Read the model definition and answer for the solid it produces. Units are mm, in the model's axes. Face numbers are marked on the shaded views. A direction names the side the tool comes from. Round coordinates to 2 decimals unless told otherwise and drop trailing zeros. Order: outer loops, then holes, each group sorted by start corner. A loop starts at its lowest first (then second) coordinate and runs counter-clockwise, first axis right, second up. Notation, with made-up numbers: (14, -24.5) -> (40, -24.5) arc R12 ccw to (40, -18.5) -> close; hole circle Ø11 at (61.25, 62). An arc over 180 degrees is marked (long way). Use a Markdown table: item, result. Add a question column.
1. For the marked faces 1 and 2, determine the directions among +Z, -Z, +X, -X, +Y, -Y from which every point of the face is accessible in a straight line to the end or side of a thin tool.
2. The mould has two halves that part along Y. Classify the marked faces 3, 4 and 5: +Y half, -Y half, draft (parallel to the pull), parting line (faces both ways), or undercut.
3. Section D-D, the plane x = -34.5 is taken. Give the vertices of the cut face in (y, z).
4. Section C-C, the plane x = -25.75 is taken. Give the vertices of the cut face in (y, z), then the cut area to 3 significant figures.
5. Given pin 1 (3 mm diameter, centred on x = -25.5, z = 389.5, fed in from -Y); pin 2 (8 mm diameter, centred on y = 15.27, z = 391.14, fed in from +X); pin 3 (6 mm diameter, centred on x = -28.5, z = 394.5, fed in from +Y); pin 4 (12 mm diameter, centred on x = -32, y = 17, fed in from +Z), each flat-ended and moving along its own axis, determine where each tip first touches the part or whether it passes through.
6. Section A-A, the plane y = 15.25 is taken. Give the vertices of the cut face in (x, z), then the cut area to 3 significant figures.
7. Section B-B, the plane z = 396 is taken. Give the vertices of the cut face in (x, y), then the cut area to 3 significant figures.
8. Consider L1, parallel to X at y = 12.75, z = 396.5; L2, parallel to Y at x = -22, z = 398.5; L3, parallel to Y at x = -36.75, z = 389.25. Determine where each line is inside the solid, lowest interval first. Write a range as [from, to].
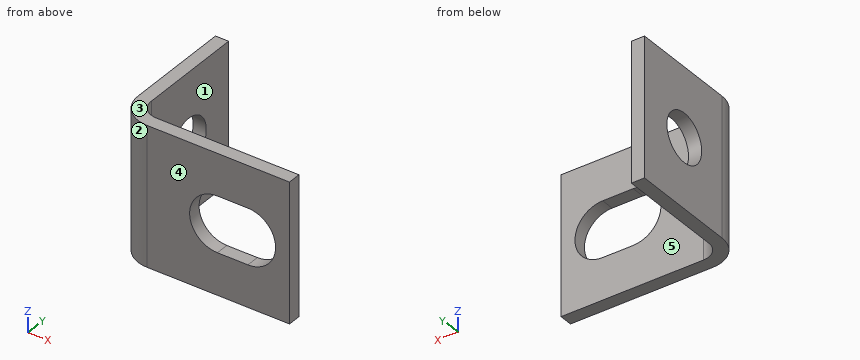
```python
from build123d import *

# Parameters (mm, degrees)
SKETCH2_W                    = 25
SKETCH2_H                    = 20
BASE_FLANGE1_DEPTH           = 1.89738
EDGE_FLANGE1_STRIP_W         = 12.66952
EDGE_FLANGE1_STRIP_H         = 1.89738
EDGE_FLANGE1_STRIP_CUT_DEPTH = 20
EDGE_FLANGE1_DEPTH           = 20
SKETCH11_R                   = 3.5
CUT_EXTRUDE1_DEPTH           = 10
CUT_EXTRUDE2_DEPTH           = 10


# Sheet-metal steps are written as plain solids
with BuildPart() as part:
    # Sketch2 → Base-Flange1 (new body)
    with BuildSketch(Plane(origin=(0, 3.26937922, 0), x_dir=(1, 0, 0), z_dir=(0, 1, 0))):
        with Locations((-25.783324161, -391.136685208)):
            Rectangle(SKETCH2_W, SKETCH2_H)
    extrude(amount=BASE_FLANGE1_DEPTH)

    # Edge-Flange1 strip (across the edge) → Edge-Flange1 strip cut (cut)
    with BuildSketch(Plane(origin=(-38.283324161, 5.16675922, 381.136685208), x_dir=(1, 0, 0), z_dir=(0, 0, 1))):
        with Locations((-1.89738, -0.94869)):
            Rectangle(EDGE_FLANGE1_STRIP_W, EDGE_FLANGE1_STRIP_H)
    extrude(amount=EDGE_FLANGE1_STRIP_CUT_DEPTH, mode=Mode.SUBTRACT)

    # Edge-Flange1 section (across the edge) → Edge-Flange1 (add)
    with BuildSketch(Plane(origin=(-38.283324161, 5.16675922, 381.136685208), x_dir=(1, 0, 0), z_dir=(0, 0, 1))):
        with BuildLine():
            Line((0, 2.54), (0, 18.10262))
            Line((0, 18.10262), (1.89738, 18.10262))
            Line((1.89738, 18.10262), (1.89738, 2.54))
            ThreePointArc((1.89738, 2.54), (2.641328776, 0.743948776), (4.43738, 0))
            Line((4.43738, 0), (4.43738, -1.89738))
            ThreePointArc((4.43738, -1.89738), (1.299678511, -0.597701489), (0, 2.54))
        make_face()
    extrude(amount=EDGE_FLANGE1_DEPTH)

    # Sketch11 → Cut-Extrude1 (cut)
    with BuildSketch(Plane.ZY.offset(38.283324161)):
        with Locations(Location((391.136685208, 15.26937922, 0), (0, 0, 270))):
            Circle(SKETCH11_R)
    extrude(amount=-CUT_EXTRUDE1_DEPTH, mode=Mode.SUBTRACT)

    # Sketch13 → Cut-Extrude2 (cut)
    with BuildSketch(Plane(origin=(0, 5.16675922, 0), x_dir=(1, 0, 0), z_dir=(0, 1, 0))):
        with BuildLine():
            Line((-23.678800395, -387.136685208), (-19.283324161, -387.136685208))
            ThreePointArc((-19.283324161, -387.136685208), (-15.283324161, -391.136685208), (-19.283324161, -395.136685208))
            Line((-19.283324161, -395.136685208), (-23.678800395, -395.136685208))
            ThreePointArc((-23.678800395, -395.136685208), (-27.678800395, -391.136685208), (-23.678800395, -387.136685208))
        make_face()
    extrude(amount=-CUT_EXTRUDE2_DEPTH, mode=Mode.SUBTRACT)


solid = part.part
```
Verdict:
| question | item | result |
|---|---|---|
| 1 | face 1 | +Z, -Z, +X, +Y |
| 1 | face 2 | +Z, -Z, -X, -Y |
| 2 | face 3 | draft |
| 2 | face 4 | -Y half |
| 2 | face 5 | +Y half |
| 3 | outline | (3.32, 381.14) -> (5.25, 381.14) -> (5.25, 401.14) -> (3.32, 401.14) -> close |
| 4 | outline | (3.27, 381.14) -> (5.17, 381.14) -> (5.17, 387.71) -> (3.27, 387.71) -> close; (3.27, 394.56) -> (5.17, 394.56) -> (5.17, 401.14) -> (3.27, 401.14) -> close |
| 4 | area | 25.0 mm2 |
| 5 | pin 1 | passes through |
| 5 | pin 2 | stops at x = -36.39 |
| 5 | pin 3 | stops at y = 5.17 |
| 5 | pin 4 | stops at z = 401.14 |
| 6 | outline | (-38.28, 381.14) -> (-36.39, 381.14) -> (-36.39, 387.64) -> (-38.28, 387.64) -> close; (-38.28, 394.64) -> (-36.39, 394.64) -> (-36.39, 401.14) -> (-38.28, 401.14) -> close |
| 6 | area | 24.7 mm2 |
| 7 | outline | (-38.28, 7.71) arc R4.44 ccw to (-33.85, 3.27) -> (-13.28, 3.27) -> (-13.28, 5.17) -> (-33.85, 5.17) arc R2.54 cw to (-36.39, 7.71) -> (-36.39, 23.27) -> (-38.28, 23.27) -> close |
| 7 | area | 78.9 mm2 |
| 8 | L1 | x = [-38.28, -36.39] |
| 8 | L2 | y = [3.27, 5.17] |
| 8 | L3 | y = [4.35, 12.32], [18.22, 23.27] |
